Source: CAD feature listing. Evaluate the final solid. Frame: model axes, mm. Coordinates: 2 decimals unless noted, no trailing zeros. Order: outer loops, then holes, each group sorted by start corner. A loop starts at its lowest first (then second) coordinate and runs counter-clockwise, first axis right, second up.
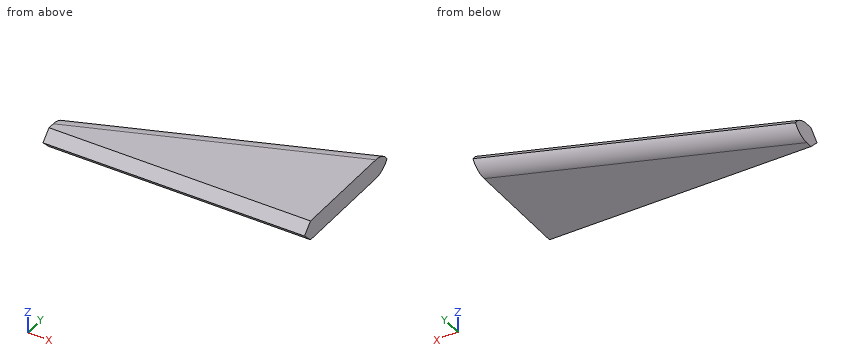
```python
from build123d import *

# Parameters (mm, degrees)
F0_W        = 66.6544139385
F0_H        = 12.0955891907
F1_DEPTH    = 5
F2_T1_DEPTH = 96.2663247468
F3_T1_DEPTH = 92.3712438182


# Not quite as in the source:
# - a fillet or chamfer that OpenCascade refuses, or shapes differently, is made with other operations: its cross-section is extruded or revolved along the edge and cut away or added


with BuildPart() as f1:
    # F0 (on Top) → F1 (new body)
    with BuildSketch(Plane.XY):
        Polygon((-33.3272069693, 6.0477945954), (33.3272069693, 6.0477945954), (33.3272069693, 31.2683843076), align=None)
        Rectangle(F0_W, F0_H)
    extrude(amount=F1_DEPTH)

    # F2: fillet of radius 5 on 2 edges, made by hand

    # F2_s2 → F2_t1 (cut)
    with BuildSketch(Plane(origin=(51.1939340465, 19.37067825, 0), x_dir=(0, 0, 1), z_dir=(-0.9352862544, -0.3538921054, 0))):
        with BuildLine():
            ThreePointArc((0, 17.4506545977), (3.5355339059, 15.9861885036), (5, 12.4506545977))
            Line((5, 12.4506545977), (5, 17.4506545977))
            Line((5, 17.4506545977), (0, 17.4506545977))
        make_face()
        with BuildLine():
            ThreePointArc((5, 17.4506545977), (1.4644660941, 15.9861885036), (0, 12.4506545977))
            Line((0, 12.4506545977), (0, 17.4506545977))
            Line((0, 17.4506545977), (5, 17.4506545977))
        make_face()
    extrude(amount=F2_T1_DEPTH, mode=Mode.SUBTRACT)

    # F3: chamfer of 5 on 2 edges, made by hand

    # F3_s2 → F3_t1 (cut)
    with BuildSketch(Plane.YZ.offset(-46.1856219091)):
        Polygon((-1.0477945954, 5), (-6.0477945954, 0), (-6.0477945954, 5), align=None)
        Polygon((-1.0477945954, 0), (-6.0477945954, 5), (-6.0477945954, 0), align=None)
    extrude(amount=F3_T1_DEPTH, mode=Mode.SUBTRACT)


solid = f1.part
```
Q1. Section query A-A on z = 1.6. Output: boundary loops of the cut face in (x, y).
Solutions:
outline: (-33.33, -2.65) - (33.33, -2.65) - (33.33, 29.84) - (-33.33, 4.62) - close
Q2. Material intervals for line 1 along Z through (x, y) = (-1, 14.5); line 2 along Y through (x, z) = (-19, 4.5); line 3 along Z through (x, y) = (4.5, 17), sorted ascending.
Solutions:
line 1: z = 0.22 to 4.78
line 2: y = -1.55 to 8.45
line 3: z = 0.36 to 4.64
Q3. Pin query (flat end, axial travel): P1, Ø2, axis at x = -2, z = 4, coming from the +Y side. Return the tip coordinate at first contact, or that it passes through.
Solutions:
P1: stops at y = 16.92
